```python
from build123d import *

# Parameters (mm, degrees)
BOSS_EXTRUDE1_DEPTH = 3
SKETCH2_R           = 4
BOSS_EXTRUDE2_DEPTH = 11
FILLET1_R           = 2
FILLET2_R           = 0.5


with BuildPart() as part:
    # Sketch1 → Boss-Extrude1 (new body)
    with BuildSketch(Plane.XY):
        Polygon((0, 10), (10, 0), (0, -10), (-10, 0), align=None)
    extrude(amount=-BOSS_EXTRUDE1_DEPTH)

    # Sketch2 → Boss-Extrude2 (add)
    with BuildSketch(Plane.XY):
        Circle(SKETCH2_R)
    extrude(amount=BOSS_EXTRUDE2_DEPTH)

    # Fillet1
    fillet1_edges = [part.edges().sort_by_distance(p)[0] for p in [
        (0, 10, -1.5),
        (10, 0, -1.5),
        (0, -10, -1.5),
        (-10, 0, -1.5),
    ]]
    fillet(fillet1_edges, radius=FILLET1_R)

    # Fillet2
    fillet2_edges = [part.edges().sort_by_distance(p)[0] for p in [
        (-4, 0, 11),
    ]]
    fillet(fillet2_edges, radius=FILLET2_R)


solid = part.part
```
For this review, take the finished solid that the model builds, in its own axes (mm). A direction names the side the tool comes from. Coordinates: 2 decimals unless noted, no trailing zeros. Write each loop counter-clockwise with the first axis right and the second up, starting at its lowest first coordinate (ties: lowest second). Pieces come first, ordered by that corner, then holes. Notation, with made-up numbers: (49.5, 61.5) - (106.5, 61.5) arc R16 cw to (106.5, 86.5) - close; hole circle Ø9 at (-30, 5.25). An arc over 180 degrees is marked (long way). Put each result on its own line as item: value.
1. Add section B-B, the plane z = -0.25. Give the boundary of the cut face in (x, y), then the cut area to 3 significant figures.
Values found:
outline: (-8.59, -1.41) - (-1.41, -8.59) arc R2 ccw to (1.41, -8.59) - (8.59, -1.41) arc R2 ccw to (8.59, 1.41) - (1.41, 8.59) arc R2 ccw to (-1.41, 8.59) - (-8.59, 1.41) arc R2 ccw to start
area: 197 mm²
2. Wall thickness on probe 1 along Z at (x, y) = (4.75, -2.5); probe 2 along Y at (x, z) = (3, 3.5); probe 3 along X at (y, z) = (-1.75, 6.5): over which ranges is each line inside the solid? List them lowest first.
Values found:
probe 1: -3 to 0
probe 2: -2.65 to 2.65
probe 3: -3.6 to 3.6
3. Add section A-A, the plane y = 0. Give the boundary of the cut face in (x, z).
Values found:
outline: (-9.17, -3) - (9.17, -3) - (9.17, 0) - (4, 0) - (4, 10.5) arc R0.5 ccw to (3.5, 11) - (-3.5, 11) arc R0.5 ccw to (-4, 10.5) - (-4, 0) - (-9.17, 0) - close
4. For pin 1 (6 mm diameter, centred on y = -6.5, z = 7.5, fed in from +X); pin 2 (1 mm diameter, centred on x = 1, z = 9, fed in from -Y); pin 3 (1 mm diameter, centred on x = -2.5, y = -4, fed in from +Z), all flat-tipped, find the tip position at first contact; note any pin that passes through.
Values found:
pin 1: x = 1.94
pin 2: y = -3.97
pin 3: z = 0
5. Add section D-D, the plane z = 8.5. Give the boundary of the cut face in (x, y).
Values found:
outline: circle Ø8 at (0, 0)
6. Machinability: for faces 1 (the flat face through (-5, 5, -1)), 2 (the cylindrical face through (-0.867, -3.905, 5.176)), which of the approach directions +Z, -Z, +X, -X, +Y, -Y give a long, thin tool a straight path to every point of the face, cutting with its end or side? Answer none if there is none.
Values found:
face 1: +Z, -Z, -X, +Y
face 2: +Z
